Model file for the job. Use its own axes, mm. Face numbers are marked on the shaded views. Round coordinates to 2 decimals unless told otherwise and drop trailing zeros. Loops run counter-clockwise (first coordinate to the right, second up) from the corner with the lowest first, then second, coordinate; pieces in that order, holes last. Notation, with made-up numbers: (-30.5, 61.25) - (-12.5, 61.25) arc R23 ccw to (-12.5, 91.25) - close; hole circle Ø3 at (-21, 46). An arc over 180 degrees is marked (long way). Answer as a JSON object with one key per item and string values.
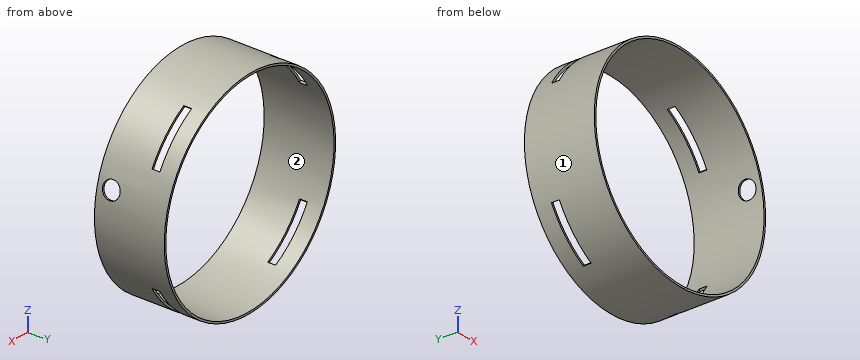
from build123d import *

# Parameters (mm, degrees)
SKETCH1_R           = 77.6224
SKETCH1_R_2         = 76.2
BOSS_EXTRUDE1_DEPTH = 25.4
SKETCH2_W           = 40.64
SKETCH2_H           = 5.715
CUT_EXTRUDE1_DEPTH  = 113.674903876
CIRPATTERN1_COUNT   = 4
SKETCH3_R           = 6.35
CUT_EXTRUDE2_DEPTH  = 6.35


with BuildPart() as part:
    # Sketch1 → Boss-Extrude1 (new, symmetric)
    with BuildSketch(Plane(origin=(0, 0, 0), x_dir=(1, 0, 0), z_dir=(0, 1, 0))):
        with Locations(Location((0, 0, 0), (0, 0, 270))):
            Circle(SKETCH1_R)
        with Locations(Location((0, 0, 0), (0, 0, 270))):
            Circle(SKETCH1_R_2, mode=Mode.SUBTRACT)
    extrude(amount=BOSS_EXTRUDE1_DEPTH, both=True)

    # Sketch2 → Cut-Extrude1 (cut, through all)
    with BuildSketch(Plane(origin=(0, 0, 0), x_dir=(0.7071067811865477, 0, 0.7071067811865475), z_dir=(-0.7071067811865475, 0, 0.7071067811865477))):
        with Locations((0, 11.1125)):
            Rectangle(SKETCH2_W, SKETCH2_H)
    cut_extrude1 = extrude(amount=-CUT_EXTRUDE1_DEPTH, mode=Mode.SUBTRACT)

    # CirPattern1: Cut-Extrude1 ×4 about axis
    cirpattern1_axis = Axis((0, 0, 0), (0, 1, 0))
    for i in range(1, CIRPATTERN1_COUNT):
        add(cut_extrude1.rotate(cirpattern1_axis, i * 360 / CIRPATTERN1_COUNT), mode=Mode.SUBTRACT)

    # Sketch3 → Cut-Extrude2 (cut)
    with BuildSketch(Plane(origin=(74.977480859, 0, 20.090155447), x_dir=(0, -1, 0), z_dir=(0.9659258262890681, 0, 0.25881904510252135))):
        with Locations(Location((15.24, 0, 0), (0, 0, 90))):
            Circle(SKETCH3_R)
    extrude(amount=-CUT_EXTRUDE2_DEPTH, mode=Mode.SUBTRACT)


solid = part.part
1) Probe probe 1 along X at (y, z) = (9, 0); probe 2 along Z at (x, y) = (50, 8); probe 3 along Z at (x, y) = (13.5, -23). List the from-to ranges inside material, lowest first.
Values follow:
{"probe 1": "-77.62 to -76.2, 76.2 to 77.62", "probe 2": "-59.37 to -57.5, 57.5 to 59.37", "probe 3": "-76.44 to -74.99, 74.99 to 76.44"}
2) Two-plate mould, pull along X, no slides. Class the marked faces 1 and 2: pulls with the +X half, pulls with the -X half, needs draft (parallel to the pull), parting line crosses it, or undercut.
Values follow:
{"face 1": "parting line crosses it", "face 2": "undercut"}
3) Slice it at C-C on x = 50. List the corners of the cut face in (y, z) (3 decimals).
Values follow:
{"outline": "(-25.4, -59.374) - (8.255, -59.374) - (8.255, -57.502) - (-25.4, -57.502) - close; (-25.4, 57.502) - (8.255, 57.502) - (8.255, 59.374) - (-25.4, 59.374) - close; (13.97, -59.374) - (25.4, -59.374) - (25.4, -57.502) - (13.97, -57.502) - close; (13.97, 57.502) - (25.4, 57.502) - (25.4, 59.374) - (13.97, 59.374) - close"}
4) Slice it at B-B on z = 0. List the corners of the cut face in (x, y).
Values follow:
{"outline": "(-77.62, -25.4) - (-76.2, -25.4) - (-76.2, 25.4) - (-77.62, 25.4) - close; (76.2, -25.4) - (77.62, -25.4) - (77.62, 25.4) - (76.2, 25.4) - close"}
5) Drop flat-ended pins along their axis: P1, Ø8, axis at y = 19.5, z = 0.5, coming from the -X side; P2, Ø1, axis at x = -36, y = 2, coming from the +Z side; P3, Ø1.5, axis at x = 14.5, y = 19, coming from the -Z side. Give the stop position or say it passes through.
Values follow:
{"P1": "x = -77.62", "P2": "z = 69.03", "P3": "z = -76.39"}
6) Slice it at A-A on x = 0. List the corners of the cut face in (y, z), then the cut area to 3 significant figures.
Values follow:
{"outline": "(-25.4, -77.62) - (25.4, -77.62) - (25.4, -76.2) - (-25.4, -76.2) - close; (-25.4, 76.2) - (25.4, 76.2) - (25.4, 77.62) - (-25.4, 77.62) - close", "area": "145 mm²"}
7) Slice it at D-D on z = 63.5. List the corners of the cut face in (x, y) (3 decimals).
Values follow:
{"outline": "(-44.643, -25.4) - (-42.121, -25.4) - (-42.121, 8.255) - (-44.643, 8.255) - close; (-44.643, 13.97) - (-42.121, 13.97) - (-42.121, 25.4) - (-44.643, 25.4) - close; (42.121, -25.4) - (44.643, -25.4) - (44.643, 8.255) - (42.121, 8.255) - close; (42.121, 13.97) - (44.643, 13.97) - (44.643, 25.4) - (42.121, 25.4) - close"}
